The listing builds one solid part. Answer for the finished solid, in the listing's coordinates (mm). A direction names the side the tool comes from. Give positions to 0.01 mm unless a question says otherwise; leave off trailing zeros. One line per item, written item: value. Start each with the question number.
Q1. A cutting plane is placed at A-A, the plane x = 16. State how many separate pieces and enclosed holes the cut face has, and give its area (3 significant figures).
Q2. The mould has two halves that part along X. Classify faces 3 (the flat face through (42, 3, 1)), 4 (the flat face through (1, 3, -9.46)), 5 (the flat face through (-26, 0, -1)), 6 (the flat face through (1, 3, -30.761)): +X half, -X half, draft (parallel to the pull), parting line (faces both ways), or undercut.
Q3. For faces 1 (the flat face through (1, 3, 11.841)), 2 (the flat face through (-26, 6.35, -1)), determine the directions among +Z, -Z, +X, -X, +Y, -Y from which every point of the face is accessible in a straight line to the end or side of a thin tool.
Q4. Flat-ended cylindrical pins translate along their axes: pin 1 (1.8 mm diameter, centred on x = -58.35, z = -63.178, fed in from +Y); pin 2 (5 mm diameter, centred on x = -52.5, z = -29.5, fed in from -Y). Find the tip coordinate at first contact, or state that the pin passes through.
from build123d import *

# Parameters (mm, degrees)
BOSS_EXTRUDE1_DEPTH       = 6.35
F_4_CLEARANCE_HOLE1_D     = 2.9464
CUT_EXTRUDE2_DEPTH        = 7.35
F_4_CLEARANCE_HOLE2_D     = 2.9464
F_4_CLEARANCE_HOLE2_DEPTH = 6.35
F_4_CLEARANCE_HOLE2_TIP   = 0.885187864


with BuildPart() as part:
    # Sketch1 → Boss-Extrude1 (new body)
    with BuildSketch(Plane(origin=(0, 0, 0), x_dir=(1, 0, 0), z_dir=(0, 1, 0))):
        Polygon((-42, -66.35), (42, -66.35), (42, 66.35), (-42, 66.35), (-92.8, 66.35), (-92.8, -66.35), align=None)
    extrude(amount=BOSS_EXTRUDE1_DEPTH)

    # #4 Clearance Hole1 (through all)
    with Locations(Plane(origin=(0, 6.35, 0), x_dir=(1, 0, 0), z_dir=(0, 1, 0))):
        with Locations((38.825, 35.997), (38.825, -35.997)):
            Hole(F_4_CLEARANCE_HOLE1_D / 2)

    # Sketch3 → Cut-Extrude2 (cut, through all)
    with BuildSketch(Plane(origin=(0, 6.35, 0), x_dir=(1, 0, 0), z_dir=(0, 1, 0))):
        with BuildLine():
            Line((-38.825, -52.85625), (38.825, -52.85625))
            ThreePointArc((38.825, -52.85625), (39.61875, -53.65), (38.825, -54.44375))
            Line((38.825, -54.44375), (-38.825, -54.44375))
            ThreePointArc((-38.825, -54.44375), (-39.61875, -53.65), (-38.825, -52.85625))
        make_face()
        with BuildLine():
            Line((-38.825, -31.555), (38.825, -31.555))
            ThreePointArc((38.825, -31.555), (39.61875, -32.34875), (38.825, -33.1425))
            Line((38.825, -33.1425), (-38.825, -33.1425))
            ThreePointArc((-38.825, -33.1425), (-39.61875, -32.34875), (-38.825, -31.555))
        make_face()
        with BuildLine():
            Line((-38.825, -10.25375), (38.825, -10.25375))
            ThreePointArc((38.825, -10.25375), (39.61875, -11.0475), (38.825, -11.84125))
            Line((38.825, -11.84125), (-38.825, -11.84125))
            ThreePointArc((-38.825, -11.84125), (-39.61875, -11.0475), (-38.825, -10.25375))
        make_face()
        with BuildLine():
            Line((-38.825, 11.0475), (38.825, 11.0475))
            ThreePointArc((38.825, 11.0475), (39.61875, 10.25375), (38.825, 9.46))
            Line((38.825, 9.46), (-38.825, 9.46))
            ThreePointArc((-38.825, 9.46), (-39.61875, 10.25375), (-38.825, 11.0475))
        make_face()
        with BuildLine():
            Line((-38.825, 32.34875), (38.825, 32.34875))
            ThreePointArc((38.825, 32.34875), (39.61875, 31.555), (38.825, 30.76125))
            Line((38.825, 30.76125), (-38.825, 30.76125))
            ThreePointArc((-38.825, 30.76125), (-39.61875, 31.555), (-38.825, 32.34875))
        make_face()
        with BuildLine():
            Line((-38.825, 53.65), (38.825, 53.65))
            ThreePointArc((38.825, 53.65), (39.61875, 52.85625), (38.825, 52.0625))
            Line((38.825, 52.0625), (-38.825, 52.0625))
            ThreePointArc((-38.825, 52.0625), (-39.61875, 52.85625), (-38.825, 53.65))
        make_face()
    extrude(amount=-CUT_EXTRUDE2_DEPTH, mode=Mode.SUBTRACT)

    # #4 Clearance Hole2
    with Locations(Plane(origin=(0, 6.35, 0), x_dir=(1, 0, 0), z_dir=(0, 1, 0))):
        with Locations((-58.35, 63.178000009), (-58.35, -63.171999991)):
            Hole(F_4_CLEARANCE_HOLE2_D / 2, depth=F_4_CLEARANCE_HOLE2_DEPTH)
            with Locations((0, 0, -(F_4_CLEARANCE_HOLE2_DEPTH + F_4_CLEARANCE_HOLE2_TIP / 2))):  # 118° drill point
                Cone(0, F_4_CLEARANCE_HOLE2_D / 2, F_4_CLEARANCE_HOLE2_TIP, mode=Mode.SUBTRACT)


solid = part.part
Answer block:
1. separate pieces: 7
1. enclosed holes: 0
1. area: 782 mm^2
2. face 3: +X half
2. face 4: undercut
2. face 5: draft
2. face 6: undercut
3. face 1: +Y, -Y
3. face 2: +Z, -Z, +X, -X, +Y
4. pin 1: through
4. pin 2: y = 0
